For this review, take the finished solid that the model builds, in its own axes (mm). Face numbers are marked on the shaded views. A direction names the side the tool comes from. Round coordinates to 2 decimals unless told otherwise and drop trailing zeros. Order: outer loops, then holes, each group sorted by start corner. A loop starts at its lowest first (then second) coordinate and runs counter-clockwise, first axis right, second up. Notation, with made-up numbers: M 9,52.25 L 50,52.25 A21 cw 50,85.25 Z; hole C 86.25,54 d2. An arc over 180 degrees is marked long. Use a Markdown table: item, result.
from build123d import *

# Parameters (mm, degrees)
BOSS_EXTRUDE1_DEPTH = 10
BOSS_EXTRUDE2_START = -14
BOSS_EXTRUDE2_DEPTH = 14
SKETCH3_W           = 20
SKETCH3_H           = 6
CUT_EXTRUDE2_DEPTH  = 73.828565824


with BuildPart() as part:
    # Sketch1 → Boss-Extrude1 (new body)
    with BuildSketch(Plane.XY):
        with BuildLine():
            ThreePointArc((22, 0), (0, 22), (-22, 0))
            Line((-22, 0), (-10, 0))
            ThreePointArc((-10, 0), (0, 10), (10, 0))
            Line((10, 0), (22, 0))
        make_face()
        with BuildLine():
            Line((-22, 0), (-22, -16))
            Line((-22, -16), (22, -16))
            Line((22, -16), (22, 0))
            Line((22, 0), (10, 0))
            ThreePointArc((10, 0), (0, -10), (-10, 0))
            Line((-10, 0), (-22, 0))
        make_face()
    extrude(amount=BOSS_EXTRUDE1_DEPTH)

    # Sketch1_3 → Boss-Extrude2 (add)
    with BuildSketch(Plane.XY.offset(BOSS_EXTRUDE2_START)):
        with BuildLine():
            Line((-22, 52), (-22, 0))
            ThreePointArc((-22, 0), (0, 22), (22, 0))
            Line((22, 0), (22, 26.596588156))
            Line((22, 26.596588156), (-22, 52))
        make_face()
        with BuildLine():
            ThreePointArc((22, 0), (0, 22), (-22, 0))
            Line((-22, 0), (-10, 0))
            ThreePointArc((-10, 0), (0, 10), (10, 0))
            Line((10, 0), (22, 0))
        make_face()
        with BuildLine():
            Line((-22, 0), (-22, -16))
            Line((-22, -16), (22, -16))
            Line((22, -16), (22, 0))
            Line((22, 0), (10, 0))
            ThreePointArc((10, 0), (0, -10), (-10, 0))
            Line((-10, 0), (-22, 0))
        make_face()
    extrude(amount=BOSS_EXTRUDE2_DEPTH)

    # Sketch3 → Cut-Extrude2 (cut, through all)
    with BuildSketch(Plane.XZ.offset(16)):
        with Locations((0, -11)):
            Rectangle(SKETCH3_W, SKETCH3_H)
    extrude(amount=-CUT_EXTRUDE2_DEPTH, mode=Mode.SUBTRACT)


solid = part.part
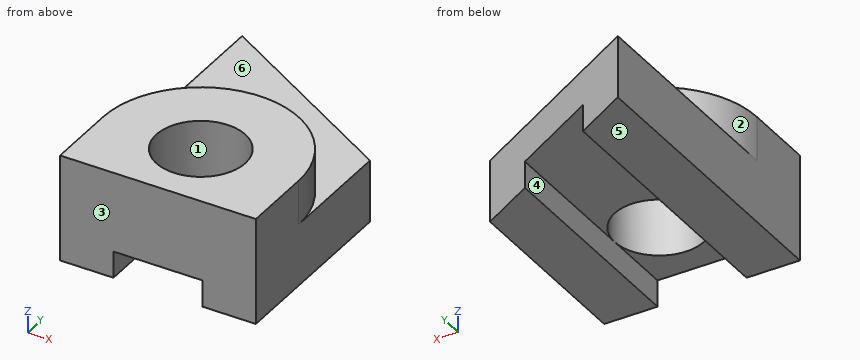
Q1. Wall thickness on line 1 along Y through (x, z) = (0, 4.75); line 2 along X through (y, z) = (-9, -10.25); line 3 along Z through (x, y) = (16, 15.5): over which ranges is each line inside the solid? List them lowest first. Write a range as [from, to].
Determined:
| item | result |
|---|---|
| line 1 | y = [-16, -10], [10, 22] |
| line 2 | x = [-22, -10], [10, 22] |
| line 3 | z = [-14, 0] |
Q2. Add section D-D (y = 5.5). Write out the cut boundary in (x, z).
Determined:
| item | result |
|---|---|
| outline | M -22,-14 L -10,-14 L -10,-8 L -8.35,-8 L -8.35,10 L -21.3,10 L -21.3,0 L -22,0 Z; M 8.35,-8 L 10,-8 L 10,-14 L 22,-14 L 22,0 L 21.3,0 L 21.3,10 L 8.35,10 Z |
Q3. Add section C-C (z = 4). Write out the cut boundary in (x, y).
Determined:
| item | result |
|---|---|
| outline | M -22,-16 L 22,-16 L 22,0 A22 ccw -22,0 Z; hole C 0,0 d20 |
Q4. Machinability: for the marked faces 4, 5 and 6, which of the approach directions +Z, -Z, +X, -X, +Y, -Y give a long, thin tool a straight path to every point of the face, cutting with its end or side? Answer none if there is none.
Determined:
| item | result |
|---|---|
| face 4 | -Z, +Y, -Y |
| face 5 | -Z, +X, -X, +Y, -Y |
| face 6 | +Z, +Y |
Q5. Add section B-B (x = -2.5). Write out the cut boundary in (y, z), then the cut area to 3 significant figures.
Determined:
| item | result |
|---|---|
| outline | M -16,-8 L -9.68,-8 L -9.68,10 L -16,10 Z; M 9.68,-8 L 40.74,-8 L 40.74,0 L 21.86,0 L 21.86,10 L 9.68,10 Z |
| area | 484 mm^2 |
Q6. Clearance check with flat-ended pins moving along their axes: pin 1 (1.5 mm diameter, centred on y = 17, z = 3.5, fed in from -X); pin 2 (6 mm diameter, centred on x = -2, y = 15, fed in from -Z); pin 3 (1 mm diameter, centred on y = 9.5, z = 7, fed in from +X). State where each tip first meets the part, or that it passes through.
Determined:
| item | result |
|---|---|
| pin 1 | stops at x = -14.83 |
| pin 2 | stops at z = -8 |
| pin 3 | stops at x = 20.07 |
Q7. Add section A-A (y = -6). Write out the cut boundary in (x, z).
Determined:
| item | result |
|---|---|
| outline | M -22,-14 L -10,-14 L -10,-8 L -8,-8 L -8,10 L -22,10 Z; M 8,-8 L 10,-8 L 10,-14 L 22,-14 L 22,10 L 8,10 Z |
Q8. Draft analysis for pull direction X (two halves, no side actions). For the marked faces 1, 2 and 3, state which applies: pulls with the +X half, pulls with the -X half, needs draft (parallel to the pull), parting line crosses it, or undercut.
Determined:
| item | result |
|---|---|
| face 1 | undercut |
| face 2 | parting line crosses it |
| face 3 | needs draft |
